```python
from build123d import *

# Parameters (mm, degrees)
SKETCH1_R           = 1
BOSS_EXTRUDE1_DEPTH = 17
CUT_EXTRUDE1_DEPTH  = 2
CUT_EXTRUDE2_DEPTH  = 3
CUT_EXTRUDE3_DEPTH  = 94.116031007
SKETCH5_R           = 2
SKETCH5_R_2         = 1
BOSS_EXTRUDE2_DEPTH = 3
FILLET1_START       = -84
FILLET1_DEPTH       = 46.103039735


with BuildPart() as part:
    # Sketch1 → Boss-Extrude1 (new body)
    with BuildSketch(Plane.XY):
        with BuildLine():
            Line((-12.561010035, 47.693103213), (-11.089724337, 53.437595852))
            Line((-11.089724337, 53.437595852), (-10.698403568, 54.965469926))
            ThreePointArc((-10.698403568, 54.965469926), (-11.120792406, 57.392279847), (-13.217767636, 58.684763351))
            Line((-13.217767636, 58.684763351), (-61.454584691, 65.227631075))
            ThreePointArc((-61.454584691, 65.227631075), (-64.658763624, 63.733229066), (-63.164361616, 60.529050133))
            Line((-63.164361616, 60.529050133), (-50.545614142, 55.937186437))
            Line((-50.545614142, 55.937186437), (-41.148452258, 52.517632588))
            Line((-41.148452258, 52.517632588), (-25.57571408, 46.850834736))
            Line((-25.57571408, 46.850834736), (-16.767387766, 43.645553554))
            ThreePointArc((-16.767387766, 43.645553554), (-14.456681284, 43.934299556), (-13.048668569, 45.789087654))
            Line((-13.048668569, 45.789087654), (-12.561010035, 47.693103213))
        make_face()
        with BuildLine():
            ThreePointArc((-23.185784758, 50.67045315), (-23.612180096, 49.851320869), (-24.527740143, 49.730736961))
            ThreePointArc((-24.527740143, 49.730736961), (-24.759389419, 51.48958543), (-23.185784758, 50.67045315))
        make_face(mode=Mode.SUBTRACT)
        with Locations((-20.777036606, 55.918720799)):
            Circle(SKETCH1_R, mode=Mode.SUBTRACT)
    extrude(amount=BOSS_EXTRUDE1_DEPTH)

    # Sketch2 → Cut-Extrude1 (cut, symmetric)
    with BuildSketch(Plane.XY.offset(8.5)):
        with BuildLine():
            Line((-24.51171166, 53.149116429), (-10.698403568, 54.965469926))
            Line((-10.698403568, 54.965469926), (-6.677815913, 55.49414911))
            Line((-6.677815913, 55.49414911), (-11.161264417, 41.454335722))
            Line((-11.161264417, 41.454335722), (-26.685784758, 44.980900868))
            Line((-26.685784758, 44.980900868), (-26.685784758, 47.009961102))
            Line((-26.685784758, 47.009961102), (-26.685784758, 50.67045315))
            ThreePointArc((-26.685784758, 50.67045315), (-26.065255063, 52.318965016), (-24.51171166, 53.149116429))
        make_face()
    extrude(amount=CUT_EXTRUDE1_DEPTH, both=True, mode=Mode.SUBTRACT)

    # Sketch3 → Cut-Extrude2 (cut)
    with BuildSketch(Plane.XY.offset(17)):
        with BuildLine():
            Line((-22.923684774, 57.200087897), (-29.137926811, 46.789494935))
            Line((-29.137926811, 46.789494935), (-12.362720011, 40.045691857))
            Line((-12.362720011, 40.045691857), (-5.826442747, 57.795582407))
            Line((-5.826442747, 57.795582407), (-16.920124342, 60.134250419))
            Line((-16.920124342, 60.134250419), (-21.697201499, 58.243220007))
            ThreePointArc((-21.697201499, 58.243220007), (-22.396717667, 57.823092942), (-22.923684774, 57.200087897))
        make_face()
    cut_extrude2 = extrude(amount=-CUT_EXTRUDE2_DEPTH, mode=Mode.SUBTRACT)

    # Mirror1: Cut-Extrude2 across plane
    add(cut_extrude2.mirror(Plane.XY.offset(8.5)), mode=Mode.SUBTRACT)

    # Sketch4 → Cut-Extrude3 (cut, through all)
    with BuildSketch(Plane.XY.offset(14)):
        Polygon((-19.714121893, 53.655932185), (-10.079835615, 58.181509414), (-11.289444582, 40.128166079), (-24.564448807, 44.84188173), (-23.812093713, 46.209067053), (-22.172973595, 49.187688427), align=None)
    extrude(amount=-CUT_EXTRUDE3_DEPTH, mode=Mode.SUBTRACT)

    # Sketch5 → Boss-Extrude2 (add)
    with BuildSketch(Plane(origin=(7.039796384, 51.900387509, 0), x_dir=(0.9909258444107709, -0.13440971273981925, 0), z_dir=(0.13440971273981922, 0.9909258444107708, 0))):
        with Locations((-21.928372674, -8.5)):
            Circle(SKETCH5_R)
        with Locations(Location((-21.928372674, -8.5, 0), (0, 0, 180))):
            Circle(SKETCH5_R_2, mode=Mode.SUBTRACT)
    extrude(amount=BOSS_EXTRUDE2_DEPTH)

    # Fillet1: read off the stored shape, not the designer's step
    # Fillet1 outline → Fillet1 (cut)
    with BuildSketch(Plane(origin=(0, 0, 0), x_dir=(0.34195538491818894, 0.939716188391715, 0), z_dir=(0.939716188391715, -0.341955384918189, 0)).offset(FILLET1_START)):
        with BuildLine():
            ThreePointArc((35.280734689, 12), (36.74520179, 15.535534913), (40.280737537, 17))
            Line((40.280737537, 17), (35.280734689, 17))
            Line((35.280734689, 17), (35.280734689, 12))
        make_face()
        with BuildLine():
            Line((35.280734689, 5), (35.280734689, 0))
            Line((35.280734689, 0), (40.280737537, 0))
            ThreePointArc((40.280737537, 0), (36.74520179, 1.464465087), (35.280734689, 5))
        make_face()
    extrude(amount=FILLET1_DEPTH, mode=Mode.SUBTRACT)


solid = part.part
```
For this review, take the finished solid that the model builds, in its own axes (mm). A direction names the side the tool comes from. Round coordinates to 2 decimals unless told otherwise and drop trailing zeros. Order: outer loops, then holes, each group sorted by start corner. A loop starts at its lowest first (then second) coordinate and runs counter-clockwise, first axis right, second up.
Q1. We need section B-B, the plane z = 15.75. Give the boundary of the cut face in (x, y), plus the area to 3 significant figures.
Findings below:
outline: (-64.81, 62.93) - (-27.59, 49.38) - (-22.92, 57.2) arc R2.5 cw to (-21.7, 58.24) - (-18.7, 59.43) - (-61.45, 65.23) arc R2.5 ccw to start
area: 297 mm2
Q2. Mouldability with a two-part tool opening along X and no side actions: class faces 5 (the cylindrical face through (-44.412, 55.305, 1.426)), 6 (the cylindrical face through (-13.6, 55.46, 8.54)), 7 (the cylindrical face through (-26.08, 52.3, 8.53)) as pulls with the +X half, pulls with the -X half, needs draft (parallel to the pull), parting line crosses it, or undercut.
Findings below:
face 5: pulls with the -X half
face 6: undercut
face 7: pulls with the +X half
Q3. Machinability: for faces 1 (the flat face through (-23, 50, 6.5)), 2 (the flat face through (-21, 54, 14)), 3 (the flat face through (-13.82, 54.73, 9.36)), 4 (the flat face through (-20.179, 58.844, 1.479)), which of the approach directions +Z, -Z, +X, -X, +Y, -Y give a long, thin tool a straight path to every point of the face, cutting with its end or side? Answer none if there is none.
Findings below:
face 1: +X, -Y
face 2: +Z, +X, -Y
face 3: +Z, -Z, -Y
face 4: -Z, +X, -Y
Q4. Wall thickness on line 1 (Z direction, x = -26.5, y = 50); line 2 (Z direction, x = -22.5, y = 53.75); line 3 (Y direction, x = -21.5, z = 10): over which ranges is each line inside the solid? List them lowest first.
Findings below:
line 1: z = 3 to 6.5, 10.5 to 14
line 2: z = 3 to 14
line 3: y = 53.55 to 55.23, 56.61 to 59.81
Q5. We need section A-A, the plane z = 3.5. Give the boundary of the cut face in (x, y), plus the area to 3 significant figures.
Findings below:
outline: (-64.07, 61.1) - (-23.7, 46.41) - (-19.71, 53.66) - (-11.29, 57.61) arc R3 ccw to (-13.22, 58.68) - (-61.45, 65.23) arc R2.5 ccw to start; hole circle Ø2 at (-24.19, 50.67); hole circle Ø2 at (-20.78, 55.92)
area: 429 mm2
Q6. Insertion check: P1, Ø4, axis at x = -20.5, y = 53, coming from the +Z side; P2, Ø8, axis at x = -21.5, y = 49, coming from the -Z side; P3, Ø4, axis at x = -26.5, z = 6.5, coming from the +Y side; P4, Ø1.2, axis at x = -24.19, y = 50.67, coming from the +Z side. Each pin has a flat end and moves straight along its axis. Give the tip position at first contact, or say it passes through.
Findings below:
P1: stops at z = 14
P2: stops at z = 3
P3: stops at y = 60.76
P4: passes through
